Verification items for this drawing (mm, ordinates from the low corner). Give positions to 0.01 mm unless a question says otherwise; leave off trailing zeros. Order: outer loops, then holes, each group sorted by start corner. A loop starts at its lowest first (then second) coordinate and runs counter-clockwise, first axis right, second up.
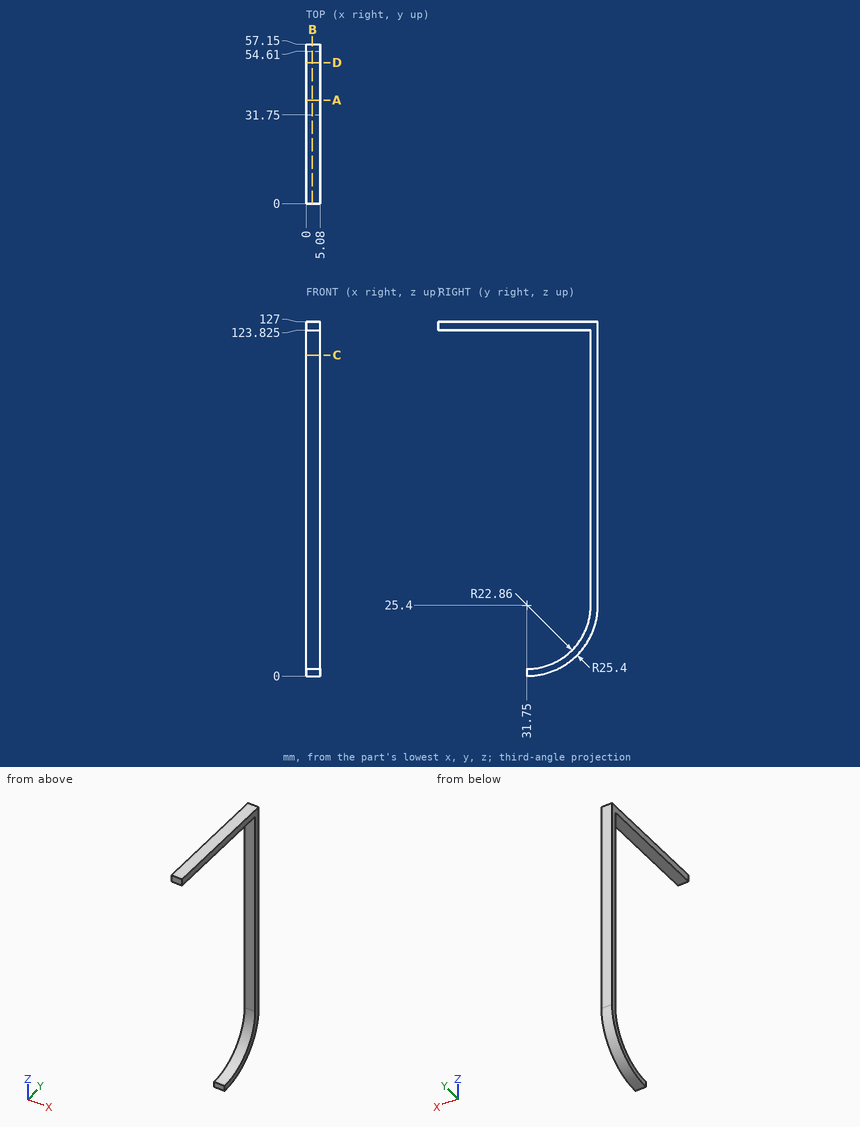
Q1. Cross-section at A-A, the plane y = 37. Record the boundary of the cut face in (x, z) (1 decimal), and give its area (3 significant figures).
Q2. Cross-section at C-C, the plane z = 115. Record the boundary of the cut face in (x, y), and give its area (3 significant figures).
Q3. Thickness scan on L1, parallel to Z at x = 1.4, y = 29 (3 decimals); L2, parallel to Y at x = 1.3, z = 25.5; L3, parallel to Z at x = 4.8, y = 39.5 (3 decimals). Record the ranges inside material, lowest first.
Q4. Cross-section at B-B, the plane x = 2.25. Record the boundary of the cut face in (y, z) (3 decimals).
Q5. Gauge pin test, flat ends, axial feed: P1, Ø2.5, axis at x = 2.5, z = 90, coming from the -Y side; P2, Ø1.3, axis at x = 3.5, z = 1.5, coming from the -Y side. Record the tip position at first contact, or that the pin passes through.
Q6. Cross-section at D-D, the plane y = 50.5. Record the boundary of the cut face in (x, z) (3 decimals), and give its area (3 significant figures).
Answers follow:
1. outline: (0, 0.5) - (5.1, 0.5) - (5.1, 3.2) - (0, 3.2) - close; (0, 123.8) - (5.1, 123.8) - (5.1, 127) - (0, 127) - close
1. area: 29.3 mm2
2. outline: (0, 54.61) - (5.08, 54.61) - (5.08, 57.15) - (0, 57.15) - close
2. area: 12.9 mm2
3. L1: z = 123.825 to 127
3. L2: y = 54.61 to 57.15
3. L3: z = 1.211 to 3.894, 123.825 to 127
4. outline: (0, 123.825) - (54.61, 123.825) - (54.61, 25.4) arc R22.86 cw to (31.75, 2.54) - (31.75, 0) arc R25.4 ccw to (57.15, 25.4) - (57.15, 127) - (0, 127) - close
5. P1: stops at y = 54.61
5. P2: stops at y = 31.75
6. outline: (0, 8.265) - (5.08, 8.265) - (5.08, 12.323) - (0, 12.323) - close; (0, 123.825) - (5.08, 123.825) - (5.08, 127) - (0, 127) - close
6. area: 36.7 mm2
